from build123d import *

# Parameters (mm, degrees)
BOSS_EXTRUDE1_DEPTH     = 1.524
CUT_EXTRUDE1_DEPTH      = 3.048
CUT_EXTRUDE1_DEPTH_BACK = 90.815491849
SKETCH2_R               = 6.35
SKETCH4_R               = 6.35
BOSS_EXTRUDE3_DEPTH     = 25.4
FILLET1_R               = 1.524


with BuildPart() as part:
    # Sketch1 → Boss-Extrude1 (new, symmetric)
    with BuildSketch(Plane.XY):
        with BuildLine():
            Line((0, 12.7), (76.2, 12.7))
            ThreePointArc((76.2, 12.7), (88.9, 0), (76.2, -12.7))
            Line((76.2, -12.7), (0, -12.7))
            ThreePointArc((0, -12.7), (-12.7, 0), (0, 12.7))
        make_face()
    extrude(amount=BOSS_EXTRUDE1_DEPTH, both=True)

    # Sketch2 → Cut-Extrude1 (cut, two sides: drawn at the far end of the back side and taken through both)
    with BuildSketch(Plane.XY.offset(-CUT_EXTRUDE1_DEPTH_BACK)):
        with Locations(Location((76.2, 0, 0), (0, 0, 180))):
            Circle(SKETCH2_R)
    extrude(amount=CUT_EXTRUDE1_DEPTH + CUT_EXTRUDE1_DEPTH_BACK, mode=Mode.SUBTRACT)

    # Sketch4 → Boss-Extrude3 (add)
    with BuildSketch(Plane.XY.offset(1.524)):
        Circle(SKETCH4_R)
    extrude(amount=BOSS_EXTRUDE3_DEPTH)

    # Fillet1
    fillet1_edges = [part.edges().sort_by_distance(p)[0] for p in [
        (88.9, 0, 1.524),
        (38.1, -12.7, 1.524),
        (-12.7, 0, 1.524),
        (88.9, 0, -1.524),
        (38.1, -12.7, -1.524),
        (-12.7, 0, -1.524),
        (38.1, 12.7, 1.524),
        (38.1, 12.7, -1.524),
    ]]
    fillet(fillet1_edges, radius=FILLET1_R - 0.0001)  # a hair under: the kernel refuses the full size


solid = part.part
Work out the finished part from the listing and answer in its coordinate system (mm). Give positions to 0.01 mm unless a question says otherwise; leave off trailing zeros. Loops run counter-clockwise (first coordinate to the right, second up) from the corner with the lowest first, then second, coordinate; pieces in that order, holes last. Notation, with made-up numbers: (-3, -10.5) -> (50, -10.5) arc R27 ccw to (50, 12.5) -> close; hole circle Ø8 at (56.25, 44). An arc over 180 degrees is marked (long way). Use a Markdown table: item, result. Add a question column.
1) Consider line 1 along Y through (x, z) = (76.2, -0.1); line 2 along Z through (x, y) = (15, 9.25); line 3 along Y through (x, z) = (76.2, 0.6). Determine where each line is inside the solid, lowest interval first.
2) Each of these flat-tipped pins is pushed along its axis until it touches: P1, Ø12, axis at y = -2, z = 21, coming from the +X side; P2, Ø1, axis at y = 5.5, z = 12.5, coming from the +X side; P3, Ø12, axis at x = 49, y = -8, coming from the +Z side. Where does it stop, or does it pass through?
3) The part is cut by section C-C, the plane z = 19.25. Determine the outline of the cut face in (x, y), plus the area to 3 significant figures.
4) For a pull along X with two mould halves and no side action, classify faces 1 (the flat face through (39, 0, 1.524)), 2 (the cylindrical face through (-1.38, -6.2, 14.05)), 3 (the cylindrical face through (82.544, -0.279, -0.021)) as +X half, -X half, draft (parallel to the pull), parting line (faces both ways), or undercut.
Reported:
| question | item | result |
|---|---|---|
| 1 | line 1 | y = -12.7 to -6.35, 6.35 to 12.7 |
| 1 | line 2 | z = -1.52 to 1.52 |
| 1 | line 3 | y = -12.58 to -6.35, 6.35 to 12.58 |
| 2 | P1 | stops at x = 6.35 |
| 2 | P2 | stops at x = 3.91 |
| 2 | P3 | stops at z = 1.52 |
| 3 | outline | circle Ø12.7 at (0, 0) |
| 3 | area | 127 mm^2 |
| 4 | face 1 | draft |
| 4 | face 2 | parting line |
| 4 | face 3 | undercut |
